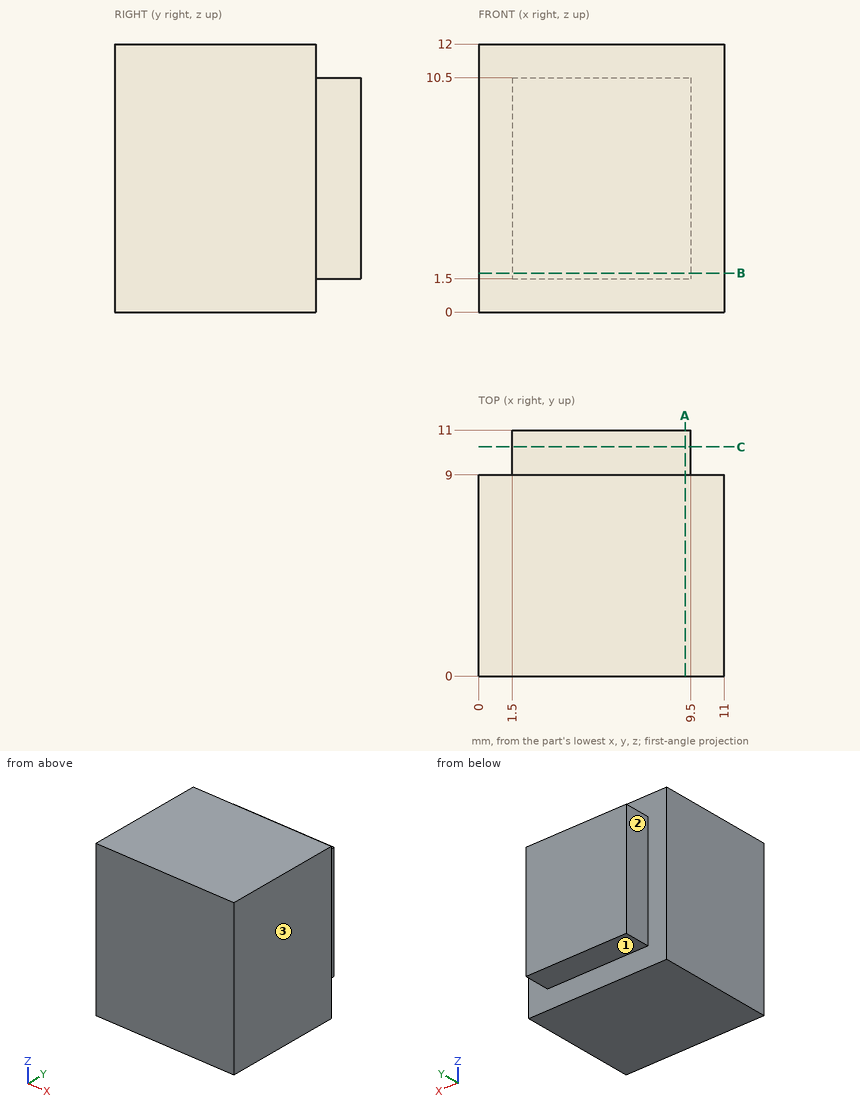
Input: dimensioned drawing with shaded views. Units: mm. Origin: part minimum x, y, z. A direction names the side the tool comes from. Give positions to 0.01 mm unless a question says otherwise; leave off trailing zeros. Loops run counter-clockwise (first coordinate to the right, second up) from the corner with the lowest first, then second, coordinate; pieces in that order, holes last. Notation, with made-up numbers: M 81,-0.75 L 127,-0.75 A16 cw 127,11.25 Z; hole C 38,45 d7. An arc over 180 degrees is marked long. Put each result on its own line as item: value.
1) Reachability of the marked faces 1, 2 and 3 from +Z, -Z, +X, -X, +Y, -Y: full face, straight path, thin tool, end or side. Return the list, or none.
Computed values:
face 1: -Z, +X, -X, +Y
face 2: +Z, -Z, -X, +Y
face 3: +Z, -Z, +X, +Y, -Y
2) Cut plane A-A, the plane x = 9.25. Return the cut outline in (y, z).
Computed values:
outline: M 0,0 L 9,0 L 9,1.5 L 11,1.5 L 11,10.5 L 9,10.5 L 9,12 L 0,12 Z
3) Material intervals for L1, parallel to X at y = 10.5, z = 7.5; L2, parallel to Y at x = 10.5, z = 7.75, sorted ascending. Write a range as from..to.
Computed values:
L1: x = 1.5..9.5
L2: y = 0..9
4) Cut plane C-C, the plane y = 10.25. Return the cut outline in (x, z).
Computed values:
outline: M 1.5,1.5 L 9.5,1.5 L 9.5,10.5 L 1.5,10.5 Z
5) Cut plane B-B, the plane z = 1.75. Return the cut outline in (x, y), plus the area to 3 significant figures.
Computed values:
outline: M 0,0 L 11,0 L 11,9 L 9.5,9 L 9.5,11 L 1.5,11 L 1.5,9 L 0,9 Z
area: 115 mm^2
6) First-contact query: P1, Ø0.6, axis at x = 7.5, y = 10, coming from the +Z side; P2, Ø1, axis at y = 10, z = 4, coming from the +X side; P3, Ø0.6, axis at x = 5, y = 10.5, coming from the -Z side. Flat tips, straight axial feed; report the tip coordinate or a pass-through.
Computed values:
P1: stops at z = 10.5
P2: stops at x = 9.5
P3: stops at z = 1.5
